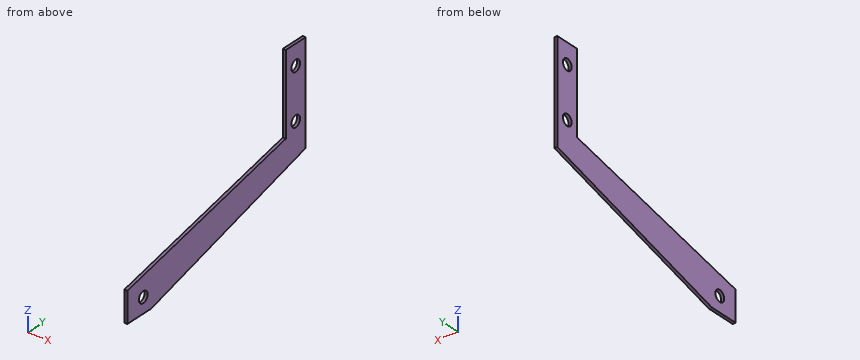
```python
from build123d import *

# Parameters (mm, degrees)
F0_R     = 5.5
F1_DEPTH = 1.5


with BuildPart() as f1:
    # F0 (on Right) → F1 (new body, symmetric)
    with BuildSketch(Plane.YZ):
        Polygon((-194.5, -55), (0, 0), (0, 100), (-25, 100), (-25, 20), (-224.5, -25), (-224.5, -55), align=None)
        with Locations((-204.5, -40)):
            Circle(F0_R, mode=Mode.SUBTRACT)
        with Locations((-12.5, 30)):
            Circle(F0_R, mode=Mode.SUBTRACT)
        with Locations((-12.5, 80)):
            Circle(F0_R, mode=Mode.SUBTRACT)
    extrude(amount=F1_DEPTH, both=True)


solid = f1.part
```
CAD build for the part. Positions are in the model's coordinates, mm. Give positions to 0.01 mm unless a question says otherwise; leave off trailing zeros. Write each loop counter-clockwise with the first axis right and the second up, starting at its lowest first coordinate (ties: lowest second). Pieces come first, ordered by that corner, then holes. Notation, with made-up numbers: M -7,39.5 L 3,39.5 A20 cw 3,76.5 Z; hole C -11.5,37.25 d3. An arc over 180 degrees is marked long. Return JSON: item names as keys, results as strings. Group by question number.
(1) Flat gauge pins, fed straight in: pin 1 Ø1 at (x, z) = (1, 73.5) entering from -Y; pin 2 Ø1.5 at (x, y) = (0, -57) entering from -Z; pin 3 Ø1.5 at (x, y) = (1, -126.5) entering from -Z. Where does each tip first touch, or does it go through?
(2) Band-saw the part on C-C (z = -40). Give the cut face in (x, y).
(3) Band-saw the part on B-B (y = -12.5). Give the cut face in (x, z), and give its area (3 significant figures).
(4) Band-saw the part on D-D (y = -204.5). Give the cut face in (x, z), and give its area (3 significant figures).
(5) Drill centre lines: L1, parallel to Z at x = 0.95, y = -12.5; L2, parallel to Z at x = -0.6, y = -204.5; L3, parallel to Z at x = 0.2, y = -10.5. Where is each one in solid material? Low to high. Write a range as [from, to].
(6) Band-saw the part on A-A (x = -0.55). Give the cut face in (y, z).
Entries:
{
 "1": {"pin 1": "stops at y = -25", "pin 2": "stops at z = -16.33", "pin 3": "stops at z = -35.98"},
 "2": {"outline": "M -1.5,-224.5 L 1.5,-224.5 L 1.5,-210 L -1.5,-210 Z; M -1.5,-199 L 1.5,-199 L 1.5,-141.45 L -1.5,-141.45 Z"},
 "3": {"outline": "M -1.5,-3.53 L 1.5,-3.53 L 1.5,24.5 L -1.5,24.5 Z; M -1.5,35.5 L 1.5,35.5 L 1.5,74.5 L -1.5,74.5 Z; M -1.5,85.5 L 1.5,85.5 L 1.5,100 L -1.5,100 Z", "area": "245 mm^2"},
 "4": {"outline": "M -1.5,-55 L 1.5,-55 L 1.5,-45.5 L -1.5,-45.5 Z; M -1.5,-34.5 L 1.5,-34.5 L 1.5,-20.49 L -1.5,-20.49 Z", "area": "70.5 mm^2"},
 "5": {"L1": "z = [-3.53, 24.5], [35.5, 74.5], [85.5, 100]", "L2": "z = [-55, -45.5], [-34.5, -20.49]", "L3": "z = [-2.97, 24.88], [35.12, 74.88], [85.12, 100]"},
 "6": {"outline": "M -224.5,-55 L -194.5,-55 L 0,0 L 0,100 L -25,100 L -25,20 L -224.5,-25 Z; hole C -204.5,-40 d11; hole C -12.5,30 d11; hole C -12.5,80 d11"}
}
